Geometry: final body of the model. Coordinates: model frame, mm. Face numbers are marked on the shaded views. A direction names the side the tool comes from. Coordinates: 2 decimals unless noted, no trailing zeros. Loops run counter-clockwise (first coordinate to the right, second up) from the corner with the lowest first, then second, coordinate; pieces in that order, holes last. Notation, with made-up numbers: (9, 85.5) -> (40, 85.5) arc R22 ccw to (40, 121.5) -> close; hole circle Ø9 at (83.5, -23). An arc over 180 degrees is marked (long way). One line per item, written item: value. Start each with the question number.
Item 1: Section query C-C on y = -21.5. Return loops of the section in (x, z), then the cut area to 3 significant figures.
Item 2: Section query B-B on x = -55.5. Return loops of the section in (y, z).
Item 3: Section query A-A on z = 7.5. Return loops of the section in (x, y).
Item 4: Section query D-D on z = 30.5. Return loops of the section in (x, y).
Item 5: Mould query, pull axis Z, two halves, no side actions, for the marked faces 3, 4 and 5. Classes: +Z half, -Z half, draft (parallel to the pull), parting line (faces both ways), or undercut.
Item 6: Contact query for flat-ended pins moving along their axis: pin 1 Ø1.5 at (y, z) = (-7.5, -8) entering from +X; pin 2 Ø12 at (x, y) = (-45, -9.5) entering from -Z; pin 3 Ø10 at (y, z) = (-15.5, 23.5) entering from -X. Output: stop coordinate, or through.
Item 7: Ray query, probe 1 along X at (y, z) = (-24.25, -1.5); probe 2 along X at (y, z) = (-17.5, -6); probe 3 along Z at (x, y) = (-64.5, -19). Return the intervals inside material, ascending. Write a range as from..to.
Item 8: Set-up query: the marked faces 1 and 2. Return all of +Z, -Z, +X, -X, +Y, -Y with unobstructed straight access to the full face (end or side cutting, diameter ignored); none if empty.
from build123d import *

# Parameters (mm, degrees)
F0_R     = 31.75
F1_DEPTH = 25.4
F2_R     = 31.75
F2_W     = 25.4
F2_H     = 38.1
F3_DEPTH = 31.242


with BuildPart() as f1:
    # F0 (on Front) → F1 (new body)
    with BuildSketch(Plane.XZ):
        with Locations((-48.727896, 9.324474)):
            Circle(F0_R)
    extrude(amount=F1_DEPTH)

    # F2 (on face) → F3 (intersect)
    with BuildSketch(Plane.XZ.offset(25.4)):
        with Locations((-48.727896, 9.324474)):
            Circle(F2_R)
        with Locations((-52.116488, 8.636362)):
            Rectangle(F2_W, F2_H, mode=Mode.SUBTRACT)
    extrude(amount=-F3_DEPTH, mode=Mode.INTERSECT)


solid = f1.part
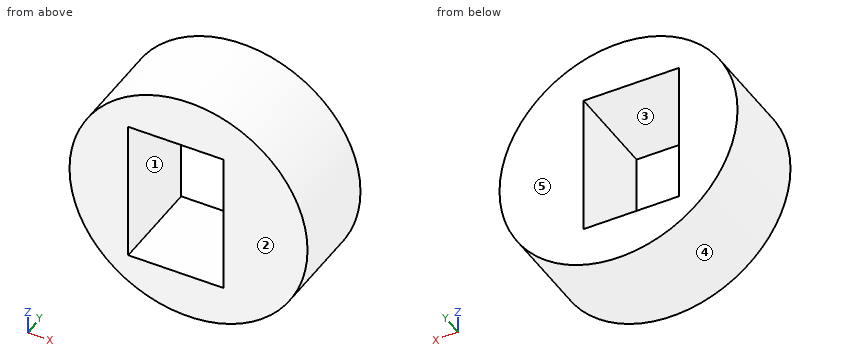
Reply:
1. outline: circle Ø63.5 at (-48.73, 9.32); hole (-64.82, -10.41) -> (-39.42, -10.41) -> (-39.42, 27.69) -> (-64.82, 27.69) -> close
1. area: 2,200 mm²
2. outline: (-25.4, -21.69) -> (0, -21.69) -> (0, -10.41) -> (-25.4, -10.41) -> close; (-25.4, 27.69) -> (0, 27.69) -> (0, 40.34) -> (-25.4, 40.34) -> close
3. outline: (-80.43, -25.4) -> (-64.82, -25.4) -> (-64.82, 0) -> (-80.43, 0) -> close; (-39.42, -25.4) -> (-17.03, -25.4) -> (-17.03, 0) -> (-39.42, 0) -> close
4. outline: (-72.39, -25.4) -> (-25.07, -25.4) -> (-25.07, 0) -> (-72.39, 0) -> close
5. face 3: undercut
5. face 4: parting line
5. face 5: draft
6. pin 1: stops at x = -21.65
6. pin 2: stops at z = -22.43
6. pin 3: stops at x = -79.12
7. probe 1: x = -78.58..-64.82, -39.42..-18.88
7. probe 2: x = -76.53..-64.82, -39.42..-20.92
7. probe 3: z = -18.23..-10.41, 27.69..36.88
8. face 1: +Y, -Y
8. face 2: +Z, -Z, +X, -X, -Y
